```python
from build123d import *

# Parameters (mm, degrees)
SKETCH1_R                                      = 32.639
SKETCH1_R_2                                    = 16.51
EXTRUDE1_DEPTH                                 = 6.35
CBORE_FOR_8_SOCKET_HEAD_CAP_SCREW1_D           = 4.9149
CBORE_FOR_8_SOCKET_HEAD_CAP_SCREW1_CBORE_D     = 7.9375
CBORE_FOR_8_SOCKET_HEAD_CAP_SCREW1_CBORE_DEPTH = 4.1656


with BuildPart() as part:
    # Sketch1 → Extrude1 (new body)
    with BuildSketch(Plane(origin=(0, 0, 0), x_dir=(1, 0, 0), z_dir=(0, 1, 0))):
        with Locations(Location((0, 0, 0), (0, 0, 270))):  # turned: the seam where the file's is
            Circle(SKETCH1_R)
        with Locations(Location((0, 0, 0), (0, 0, 270))):  # turned: the seam where the file's is
            Circle(SKETCH1_R_2, mode=Mode.SUBTRACT)
    extrude(amount=EXTRUDE1_DEPTH)

    # CBORE for #8 Socket Head Cap Screw1 (through all)
    with Locations(Plane(origin=(-18.858537854, 0, 18.858537854), x_dir=(0, 0, -1), z_dir=(0, -1, 0))):
        with Locations((0, 0), (0, 37.717075708), (37.717075708, 37.717075708), (37.717075708, 0)):
            CounterBoreHole(CBORE_FOR_8_SOCKET_HEAD_CAP_SCREW1_D / 2, CBORE_FOR_8_SOCKET_HEAD_CAP_SCREW1_CBORE_D / 2, CBORE_FOR_8_SOCKET_HEAD_CAP_SCREW1_CBORE_DEPTH)


solid = part.part
```
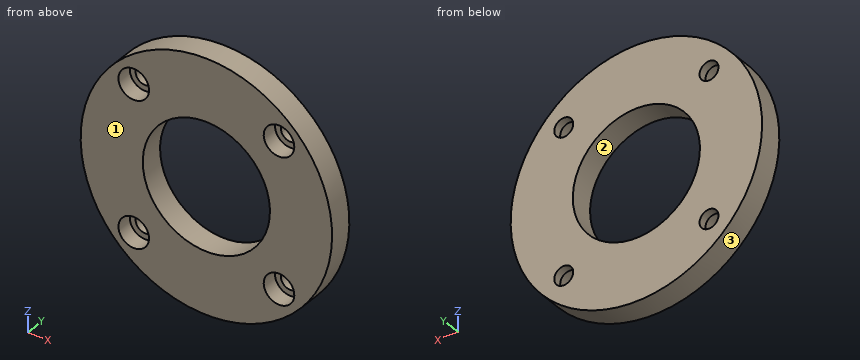
Check sheet for the modelled part. Datum: model origin and axes. Units: mm. Face numbers are marked on the shaded views. Round coordinates to 2 decimals unless told otherwise and drop trailing zeros. Order: outer loops, then holes, each group sorted by start corner. A loop starts at its lowest first (then second) coordinate and runs counter-clockwise, first axis right, second up. Notation, with made-up numbers: (-30, 71.5) -> (-26, 71.5) arc R7 cw to (-26, 83.5) -> close; hole circle Ø8 at (69.25, -13.75). An arc over 180 degrees is marked (long way). One line per item, written item: value. Start each with the question number.
Q1. Cross-section at B-B (z = 0). Record the boundary of the cut face in (x, y), and give its area (3 significant figures).
Q2. Mould release check, pull along Z, two halves, no side actions. Record for the marked faces 1, 2 and 3: pulls with the +Z half, pulls with the -Z half, needs draft (parallel to the pull), parting line crosses it, or undercut.
Q3. Cross-section at C-C (z = 18.5). Record the boundary of the cut face in (x, y), and give its area (3 significant figures).
Q4. Thickness scan on line 1 (X direction, y = 5.5, z = -20); line 2 (X direction, y = 5.5, z = -18); line 3 (X direction, y = 3, z = 0). Record the ranges inside material, lowest first.
Q5. Gauge pin test, flat ends, axial feed: pin 1 Ø6.5 at (x, z) = (18.86, -18.86) entering from -Y; pin 2 Ø6.5 at (x, z) = (-18, -20) entering from -Y; pin 3 Ø3 at (x, z) = (-18.86, -18.86) entering from -Y; pin 4 Ø2 at (y, z) = (4.5, -18) entering from +X. Record the tip position at first contact, or that the pin passes through.
Q6. Cross-section at A-A (x = 0). Record the boundary of the cut face in (y, z).
Q7. Cross-section at D-D (y = 0.75). Record the boundary of the cut face in (x, z), and give its area (3 significant figures).
Completed:
1. outline: (-32.64, 0) -> (-16.51, 0) -> (-16.51, 6.35) -> (-32.64, 6.35) -> close; (16.51, 0) -> (32.64, 0) -> (32.64, 6.35) -> (16.51, 6.35) -> close
1. area: 205 mm²
2. face 1: needs draft
2. face 2: undercut
2. face 3: parting line crosses it
3. outline: (-26.89, 0) -> (-22.81, 0) -> (-22.81, 4.17) -> (-21.29, 4.17) -> (-21.29, 6.35) -> (-26.89, 6.35) -> close; (-16.43, 4.17) -> (-14.91, 4.17) -> (-14.91, 0) -> (14.91, 0) -> (14.91, 4.17) -> (16.43, 4.17) -> (16.43, 6.35) -> (-16.43, 6.35) -> close; (21.29, 4.17) -> (22.81, 4.17) -> (22.81, 0) -> (26.89, 0) -> (26.89, 6.35) -> (21.29, 6.35) -> close
3. area: 254 mm²
4. line 1: x = -25.79 to -21.03, -16.68 to 16.68, 21.03 to 25.79
4. line 2: x = -27.23 to -21.16, -16.56 to 16.56, 21.16 to 27.23
4. line 3: x = -32.64 to -16.51, 16.51 to 32.64
5. pin 1: stops at y = 4.17
5. pin 2: stops at y = 0
5. pin 3: passes through
5. pin 4: stops at x = 27.86
6. outline: (0, -32.64) -> (6.35, -32.64) -> (6.35, -16.51) -> (0, -16.51) -> close; (0, 16.51) -> (6.35, 16.51) -> (6.35, 32.64) -> (0, 32.64) -> close
7. outline: circle Ø65.28 at (0, 0); hole circle Ø7.94 at (-18.86, -18.86); hole circle Ø7.94 at (-18.86, 18.86); hole circle Ø33.02 at (0, 0); hole circle Ø7.94 at (18.86, -18.86); hole circle Ø7.94 at (18.86, 18.86)
7. area: 2,290 mm²
